from build123d import *

# Parameters (mm, degrees)
SKETCH1_R               = 2.125
BOSS_EXTRUDE1_DEPTH     = 2
BOSS_EXTRUDE3_DEPTH     = 2
SKETCH4_R               = 2.025
CUT_EXTRUDE1_DEPTH      = 1
CUT_EXTRUDE1_DEPTH_BACK = 3
SKETCH6_R               = 2.525
BOSS_EXTRUDE4_DEPTH     = 2
FILLET1_R               = 2.5


with BuildPart() as part:
    # Sketch1 → Boss-Extrude1 (new body)
    with BuildSketch(Plane(origin=(0, 0, 0), x_dir=(1, 0, 0), z_dir=(0, 1, 0))):
        with BuildLine():
            Line((-37.655823606, 28.125414637), (-49.673639651, 37.101610798))
            ThreePointArc((-49.673639651, 37.101610798), (-59.88740123, 16.046780796), (-61.569439235, -7.294117647))
            Line((-61.569439235, -7.294117647), (-46.673607162, -5.529411765))
            ThreePointArc((-46.673607162, -5.529411765), (-45.398513836, 12.16449512), (-37.655823606, 28.125414637))
        make_face()
        with Locations((-44.167295593, 25.5)):
            Circle(SKETCH1_R, mode=Mode.SUBTRACT)
        with Locations((-51.095498823, 29.5)):
            Circle(SKETCH1_R, mode=Mode.SUBTRACT)
        with Locations((-59, 0)):
            Circle(SKETCH1_R, mode=Mode.SUBTRACT)
        with Locations((-51, 0)):
            Circle(SKETCH1_R, mode=Mode.SUBTRACT)
    extrude(amount=BOSS_EXTRUDE1_DEPTH)

    # Sketch3 → Boss-Extrude3 (add)
    with BuildSketch(Plane(origin=(0, 0, 0), x_dir=(1, 0, 0), z_dir=(0, 1, 0))):
        with BuildLine():
            Line((-70.222891931, 15.897969958), (-60.469712497, 13.689918575))
            ThreePointArc((-60.469712497, 13.689918575), (-59.670365878, 16.835897245), (-58.707466934, 19.93572989))
            Line((-58.707466934, 19.93572989), (-68.176413213, 23.151170195))
            ThreePointArc((-68.176413213, 23.151170195), (-69.294618439, 19.551364542), (-70.222891931, 15.897969958))
        make_face()
    extrude(amount=BOSS_EXTRUDE3_DEPTH)

    # Sketch4 → Cut-Extrude1 (cut, two sides)
    with BuildSketch(Plane(origin=(0, 2, 0), x_dir=(1, 0, 0), z_dir=(0, 1, 0))) as cut_extrude1_sk:
        with Locations((-64.482492158, 18.193630893)):
            Circle(SKETCH4_R)
    extrude(amount=CUT_EXTRUDE1_DEPTH, mode=Mode.SUBTRACT)
    extrude(cut_extrude1_sk.sketch, amount=-CUT_EXTRUDE1_DEPTH_BACK, mode=Mode.SUBTRACT)

    # Sketch6 → Boss-Extrude4 (add)
    with BuildSketch(Plane(origin=(0, 0, 0), x_dir=(1, 0, 0), z_dir=(0, 1, 0))):
        with BuildLine():
            Line((-61.569439235, -7.294117647), (-81.430548666, -9.647058824))
            ThreePointArc((-81.430548666, -9.647058824), (-81.961477421, -2.513208901), (-81.868629843, 4.639768059))
            Line((-81.868629843, 4.639768059), (-61.900671345, 3.508117313))
            ThreePointArc((-61.900671345, 3.508117313), (-61.970873172, -1.90023112), (-61.569439235, -7.294117647))
        make_face()
        with Locations((-76.963826359, -2.359964456)):
            Circle(SKETCH6_R, mode=Mode.SUBTRACT)
        with Locations((-66.968524234, -2.053475565)):
            Circle(SKETCH6_R, mode=Mode.SUBTRACT)
    extrude(amount=BOSS_EXTRUDE4_DEPTH)

    # Fillet1
    fillet1_edges = [part.edges().sort_by_distance(p)[0] for p in [
        (-60.469712497, 1, -13.689918575),
        (-70.222891931, 1, -15.897969958),
        (-81.430548666, 1, 9.647058824),
        (-81.868629843, 1, -4.639768059),
        (-61.900671345, 1, -3.508117313),
        (-46.673607162, 1, 5.529411765),
        (-49.673639651, 1, -37.101610798),
        (-37.655823606, 1, -28.125414637),
    ]]
    fillet(fillet1_edges, radius=FILLET1_R)


solid = part.part
For this review, take the finished solid that the model builds, in its own axes (mm). A direction names the side the tool comes from. Coordinates: 2 decimals unless noted, no trailing zeros. Order: outer loops, then holes, each group sorted by start corner. A loop starts at its lowest first (then second) coordinate and runs counter-clockwise, first axis right, second up. Notation, with made-up numbers: (-17.75, 35.5) - (11.25, 35.5) arc R18 cw to (11.25, 44.5) - close; hole circle Ø2 at (79.25, 80). An arc over 180 degrees is marked (long way). Use one line per item in the form item = value.
Q1. Consider section B-B (z = -25.5). Give the boundary of the cut face in (x, y).
Checked values:
outline = (-56.51, 0) - (-46.29, 0) - (-46.29, 2) - (-56.51, 2) - close; (-42.04, 0) - (-39.48, 0) - (-39.48, 2) - (-42.04, 2) - close
Q2. For P1, Ø3, axis at x = -76.96, z = 2.36, coming from the +Y side; P2, Ø1, axis at x = -57.5, y = 0.5, coming from the +Z side, all flat-tipped, find the tip position at first contact; note any pin that passes through.
Checked values:
P1 = through
P2 = 6.87
Q3. For probe 1 along X at (y, z) = (0.8, 3); probe 2 along Z at (x, y) = (-65, 0.95); probe 3 along X at (y, z) = (0.25, -1.5), list the stretches that pass through material, from the lowest coordinate up. Write a range as from..to.
Checked values:
probe_1 = -81.95..-79.41, -74.52..-69.31, -64.63..-46.9
probe_2 = -22.07..-20.15, -16.24..-14.72, -3.68..0.47, 3.63..7.7
probe_3 = -81.99..-60.51, -57.49..-52.51, -49.49..-46.98
Q4. For faces 4 (the flat face through (-65.33, 0.99, -14.79)), 5 (the flat face through (-63.376, 0.986, -21.521)), 6 (the flat face through (-71.946, 0.986, -4.077)), 7 (the flat face through (-60, 2, -9)), 8 (the cylindrical face through (-68.92, 0.99, -20.83)), list the 3-axis set-ups (+Z, -Z, +X, -X, +Y, -Y) from which the entire face can be reached by the end or side of a thin tool; tool diameter is ignored.
Checked values:
face_4 = -X, +Y, -Y
face_5 = -Z, +Y, -Y
face_6 = +Y, -Y
face_7 = +Z, -Z, +X, -X, +Y
face_8 = -Z, -X, +Y, -Y
Q5. Consider section C-C (z = -8.5). Give the boundary of the cut face in (x, y) (3 decimals), then the cut area to 3 significant figures.
Checked values:
outline = (-61.415, 0) - (-46.225, 0) - (-46.225, 2) - (-61.415, 2) - close
area = 30.4 mm2
Q6. Draft analysis for pull direction Z (two halves, no side actions). For faces 1 (the cylindrical face through (-80.76, 1.01, 8.82)), 2 (the cylindrical face through (-61.31, 1.014, -13.145)), 3 (the cylindrical face through (-55.41, 0.99, -27.82)), state which applies: +Z half, -Z half, draft (parallel to the pull), parting line (faces both ways), or undercut.
Checked values:
face_1 = +Z half
face_2 = undercut
face_3 = -Z half
Q7. Consider section A-A (y = 1.55). Give the number of separate pieces and of enclosed holes in the cut face, then the cut area to 3 significant figures.
Checked values:
separate_pieces = 1
enclosed_holes = 7
area = 827 mm2
